Autodesk Inventor part; units mm, degrees
ref_plane "YZ Plane" through (0, 0, 0) normal (1, 0, 0) x (0, 1, 0)
ref_plane "XZ Plane" through (0, 0, 0) normal (0, 1, 0) x (-1, 0, 0)
ref_plane "XY Plane" through (0, 0, 0) normal (0, 0, 1) x (1, 0, 0)
sketch "Sketch1" plane through (0, 0, 0) normal (0, 0, 1) x (1, 0, 0)
  line L0 (0, 8.7149) -> (0, -8.7149) construction
  line L1 (-12.4402, 0) -> (12.4402, 0) construction
  line L2 (-20, 14) -> (20, 14) construction
  line L3 (20, 14) -> (20, -14) construction
  line L4 (20, -14) -> (-20, -14) construction
  line L5 (-20, -14) -> (-20, 14) construction
  line L6 (-6, 1.25) -> (-2, 1.25)
  line L7 (-2, 1.25) -> (-2, -1.25)
  line L8 (-2, -1.25) -> (-6, -1.25)
  line L9 (-6, -1.25) -> (-6, 1.25)
  line L10 (2, 1.25) -> (6, 1.25)
  line L11 (6, 1.25) -> (6, -1.25)
  line L12 (6, -1.25) -> (2, -1.25)
  line L13 (2, -1.25) -> (2, 1.25)
  line L14 (-20, 14) -> (-20, 16)
  line L15 (-20, 16) -> (-18, 16)
  line L16 (-18, 16) -> (-18, 14)
  line L17 (-16, 14) -> (-16, 16)
  line L18 (-16, 16) -> (-14, 16)
  line L19 (-14, 16) -> (-14, 14)
  line L20 (-12, 14) -> (-12, 16)
  line L21 (-12, 16) -> (-10, 16)
  line L22 (-10, 16) -> (-10, 14)
  line L23 (-8, 14) -> (-8, 16)
  line L24 (-8, 16) -> (-6, 16)
  line L25 (-6, 16) -> (-6, 14)
  line L26 (-4, 14) -> (-4, 16)
  line L27 (-4, 16) -> (-2, 16)
  line L28 (-2, 16) -> (-2, 14)
  line L29 (0, 14) -> (0, 16)
  line L30 (0, 16) -> (2, 16)
  line L31 (2, 16) -> (2, 14)
  line L32 (4, 14) -> (4, 16)
  line L33 (4, 16) -> (6, 16)
  line L34 (6, 16) -> (6, 14)
  line L35 (8, 14) -> (8, 16)
  line L36 (8, 16) -> (10, 16)
  line L37 (10, 16) -> (10, 14)
  line L38 (12, 14) -> (12, 16)
  line L39 (12, 16) -> (14, 16)
  line L40 (14, 16) -> (14, 14)
  line L41 (16, 14) -> (16, 16)
  line L42 (16, 16) -> (18, 16)
  line L43 (18, 16) -> (18, 14)
  line L44 (-10, 14) -> (-8, 14)
  line L45 (-14, 14) -> (-12, 14)
  line L46 (-18, 14) -> (-16, 14)
  line L47 (-6, 14) -> (-4, 14)
  line L48 (-2, 14) -> (0, 14)
  line L49 (2, 14) -> (4, 14)
  line L50 (6, 14) -> (8, 14)
  line L51 (10, 14) -> (12, 14)
  line L52 (14, 14) -> (16, 14)
  line L53 (-20, -14) -> (-20, -16)
  line L54 (-20, -16) -> (-18, -16)
  line L55 (-18, -16) -> (-18, -14)
  line L56 (-16, -14) -> (-16, -16)
  line L57 (-14, -16) -> (-14, -14)
  line L58 (-16, -16) -> (-14, -16)
  line L59 (-12, -14) -> (-12, -16)
  line L60 (-10, -16) -> (-10, -14)
  line L61 (-12, -16) -> (-10, -16)
  line L62 (-8, -14) -> (-8, -16)
  line L63 (-6, -16) -> (-6, -14)
  line L64 (-8, -16) -> (-6, -16)
  line L65 (-4, -14) -> (-4, -16)
  line L66 (-2, -16) -> (-2, -14)
  line L67 (-4, -16) -> (-2, -16)
  line L68 (0, -14) -> (0, -16)
  line L69 (2, -16) -> (2, -14)
  line L70 (0, -16) -> (2, -16)
  line L71 (4, -14) -> (4, -16)
  line L72 (6, -16) -> (6, -14)
  line L73 (4, -16) -> (6, -16)
  line L74 (8, -14) -> (8, -16)
  line L75 (10, -16) -> (10, -14)
  line L76 (8, -16) -> (10, -16)
  line L77 (12, -14) -> (12, -16)
  line L78 (14, -16) -> (14, -14)
  line L79 (12, -16) -> (14, -16)
  line L80 (16, -14) -> (16, -16)
  line L81 (18, -16) -> (18, -14)
  line L82 (16, -16) -> (18, -16)
  line L83 (-18, -14) -> (-16, -14)
  line L84 (-14, -14) -> (-12, -14)
  line L85 (-10, -14) -> (-8, -14)
  line L86 (-6, -14) -> (-4, -14)
  line L87 (-2, -14) -> (0, -14)
  line L88 (2, -14) -> (4, -14)
  line L89 (6, -14) -> (8, -14)
  line L90 (10, -14) -> (12, -14)
  line L91 (14, -14) -> (16, -14)
  line L92 (18, -14) -> (20, -14)
  line L93 (18, 14) -> (20, 14)
  line L94 (20, 14) -> (20, -14)
  line L95 (-20, 14) -> (-20, -14)
  point P0 (0, 0)
  point P1 (0, 0)
  dimension "d0" = 4
  dimension "d1" = 4
  dimension "d2" = 4
  dimension "d3" = 2.5
  dimension "d4" = 28
  dimension "d5" = 40
  dimension "d10" = 2
  dimension "d11" = 2
  dimension "d14" = 4
  dimension "d19" = 2
  dimension "d22" = 4
extrude "Extrusion1" add sketch "Sketch1" along normal mid plane 2.5
properties part number "pitahaya4"
Can you work these out from the model? Positions are in its coordinate system, mm. A direction names the side the tool comes from. Coordinates: 2 decimals unless noted, no trailing zeros. Loops run counter-clockwise (first coordinate to the right, second up) from the corner with the lowest first, then second, coordinate; pieces in that order, holes last. Notation, with made-up numbers: (-21.5, 15.5) - (-9.5, 15.5) arc R10 ccw to (-9.5, 29.5) - close; hole circle Ø10 at (18.25, -10.5). An arc over 180 degrees is marked (long way). Answer as a JSON object with one key per item and string values. Group by question number.
Item 1: On a 3-axis mill with a long thin cutter (end or side, diameter ignored), from which of +Z, -Z, +X, -X, +Y, -Y can I reach the whole of each face in a straight line? I mean faces 1 (the face through (-5, -14, 0)), 2 (the face through (13, 16, 0)), 3 (the face through (-1, 14, 0)), 4 (the face through (19, -14, 0)). Say none if no direction works.
Item 2: If we section it at B-B (z = 0.85): State how many separate pieces and enclosed holes the cut face has, plus the area to 3 significant figures.
Item 3: If we mould it in two halves opening along Y, with no side actions, what happens to faces 5 (the face through (-15, -16, 0)), 6 (the face through (-14, 15, 0)), 7 (the face through (-4, -1.25, 0)), 8 (the face through (6, 0, 0))? For each: released by +Y, released by -Y, zero draft, split by the parting line, or undercut.
Item 4: If we section it at A-A (x = 3): List the corners of the cut face in (y, z) for me, plus the area to 4 significant figures.
Item 5: If we section it at C-C (x = -8.5): List the corners of the cut face in (y, z) for me.
Item 6: For pin 1 (0.6 mm diameter, centred on y = 14.5, z = 0, fed in from +X); pin 2 (0.6 mm diameter, centred on x = -0.5, z = -0.5, fed in from +Y), each with a flat end and sliding along its axis, tell me the tip position at first contact or that it passes through.
Item 7: If I drill on L1, parallel to X at y = 1, z = -1.05; L2, parallel to Y at x = -5.5, z = 0.3; L3, parallel to Y at x = 14.5, z = -0.8, over which ranges is the centre line in solid material (lowest first)? Write a range as from..to.
Returned:
{
 "1": {"face 1": "+Z, -Z, -Y", "face 2": "+Z, -Z, +X, -X, +Y", "face 3": "+Z, -Z, +Y", "face 4": "+Z, -Z, +X, -Y"},
 "2": {"separate pieces": "1", "enclosed holes": "2", "area": "1,180 mm²"},
 "3": {"face 5": "released by -Y", "face 6": "zero draft", "face 7": "undercut", "face 8": "undercut"},
 "4": {"outline": "(-14, -1.25) - (-1.25, -1.25) - (-1.25, 1.25) - (-14, 1.25) - close; (1.25, -1.25) - (14, -1.25) - (14, 1.25) - (1.25, 1.25) - close", "area": "63.75 mm²"},
 "5": {"outline": "(-14, -1.25) - (14, -1.25) - (14, 1.25) - (-14, 1.25) - close"},
 "6": {"pin 1": "stops at x = 18", "pin 2": "stops at y = 14"},
 "7": {"L1": "x = -20..-6, -2..2, 6..20", "L2": "y = -14..-1.25, 1.25..14", "L3": "y = -14..14"}
}
